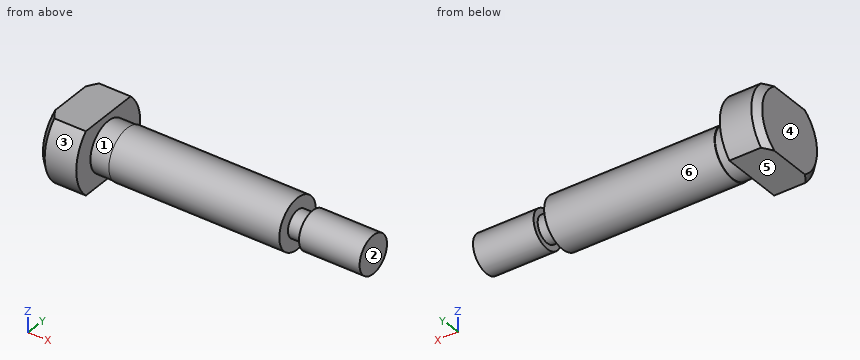
from build123d import *

# Parameters (mm, degrees)
CUT_EXTRUDE1_DEPTH      = 22.57544901
CUT_EXTRUDE1_DEPTH_BACK = 22.57544901
SKETCH2_W               = 3
SKETCH2_H               = 1
CHAMFER1_SIZE           = 0.5


with BuildPart() as part:
    # Sketch1 → Revolve1 (revolve)
    with BuildSketch(Plane.XY, mode=Mode.PRIVATE) as revolve1_sk:
        Polygon((-3, 0), (-3, 3.5), (0, 3.5), (0, 1.95), (1.5, 1.95), (1.5, 2), (15, 2), (15, 1.05), (16.2, 1.05), (16.2, 1.5), (21, 1.5), (21, 0), align=None)
    revolve(revolve1_sk.sketch.rotate(Axis((0, 0, 0), (1, 0, 0)), 90), axis=Axis((0, 0, 0), (1, 0, 0)))

    # Sketch2 → Cut-Extrude1 (cut, two sides: drawn at the far end of the back side and taken through both)
    with BuildSketch(Plane(origin=(0, 0, 0), x_dir=(1, 0, 0), z_dir=(0, 1, 0)).offset(-CUT_EXTRUDE1_DEPTH_BACK)):
        with Locations((-1.5, 3)):
            Rectangle(SKETCH2_W, SKETCH2_H)
        with Locations((-1.5, -3)):
            Rectangle(SKETCH2_W, SKETCH2_H)
    extrude(amount=CUT_EXTRUDE1_DEPTH + CUT_EXTRUDE1_DEPTH_BACK, mode=Mode.SUBTRACT)

    # Chamfer1
    chamfer1_edges = [part.edges().sort_by_distance(p)[0] for p in [
        (-3, -3.5, 0),
        (-3, 3.5, 0),
    ]]
    chamfer(chamfer1_edges, length=CHAMFER1_SIZE)


solid = part.part
The listing builds one solid part. Answer for the finished solid, in the listing's coordinates (mm). Face numbers are marked on the shaded views. A direction names the side the tool comes from. Coordinates: 2 decimals unless noted, no trailing zeros. Write each loop counter-clockwise with the first axis right and the second up, starting at its lowest first coordinate (ties: lowest second). Pieces come first, ordered by that corner, then holes. Notation, with made-up numbers: M 74.5,1.25 L 111.5,1.25 A19 cw 111.5,10.25 Z; hole C 76,28.5 d5. An arc over 180 degrees is marked long. Use one line per item in the form item = value.
Item 1: For the marked faces 5 and 6, determine the directions among +Z, -Z, +X, -X, +Y, -Y from which every point of the face is accessible in a straight line to the end or side of a thin tool.
Model answer:
face_5 = -Z, +X, -X, +Y, -Y
face_6 = +X
Item 2: Given P1, Ø2, axis at x = 4.5, z = -1, coming from the -Y side; P2, Ø1.5, axis at x = 12, y = -2, coming from the +Z side; P3, Ø3, axis at x = 14.5, z = -1, coming from the +Y side, each flat-ended and moving along its own axis, determine where each tip first touches the part or whether it passes through.
Model answer:
P1 = -2
P2 = 1.56
P3 = 2
Item 3: Find section B-B, the plane z = 0. Give the vertices of the cut face in (x, y), plus the area to 3 significant figures.
Model answer:
outline = M -3,-3 L -2.5,-3.5 L 0,-3.5 L 0,-1.95 L 1.5,-1.95 L 1.5,-2 L 15,-2 L 15,-1.05 L 16.2,-1.05 L 16.2,-1.5 L 21,-1.5 L 21,1.5 L 16.2,1.5 L 16.2,1.05 L 15,1.05 L 15,2 L 1.5,2 L 1.5,1.95 L 0,1.95 L 0,3.5 L -2.5,3.5 L -3,3 Z
area = 97.5 mm2
Item 4: Find section C-C, the plane x = 15.75. Give the vertices of the cut face in (y, z).
Model answer:
outline = C 0,0 d2.1
Item 5: The mould has two halves that part along X. Classify the marked faces 1, 2, 3 and 4: released by +X, released by -X, zero draft, split by the parting line, or undercut.
Model answer:
face_1 = undercut
face_2 = released by +X
face_3 = zero draft
face_4 = released by -X
Item 6: Find section D-D, the plane x = 0.75. Give the vertices of the cut face in (y, z).
Model answer:
outline = C 0,0 d3.9
Item 7: Find section A-A, the plane y = 0. Give the vertices of the cut face in (x, z).
Model answer:
outline = M -3,-2.5 L 0,-2.5 L 0,-1.95 L 1.5,-1.95 L 1.5,-2 L 15,-2 L 15,-1.05 L 16.2,-1.05 L 16.2,-1.5 L 21,-1.5 L 21,1.5 L 16.2,1.5 L 16.2,1.05 L 15,1.05 L 15,2 L 1.5,2 L 1.5,1.95 L 0,1.95 L 0,2.5 L -3,2.5 Z
Item 8: Find the intervals of material crossed by probe 1 along X at (y, z) = (0.5, -1.25); probe 2 along Y at (x, z) = (13.75, 0.1); probe 3 along X at (y, z) = (2.75, 0.65), in increasing order.
Model answer:
probe_1 = -3 to 15, 16.2 to 21
probe_2 = -2 to 2
probe_3 = -3 to 0
